Geometry check sheet. Reference: the model listing, model coordinates, mm. Face numbers are marked on the shaded views. Round coordinates to 2 decimals unless told otherwise and drop trailing zeros. Order: outer loops, then holes, each group sorted by start corner. A loop starts at its lowest first (then second) coordinate and runs counter-clockwise, first axis right, second up.
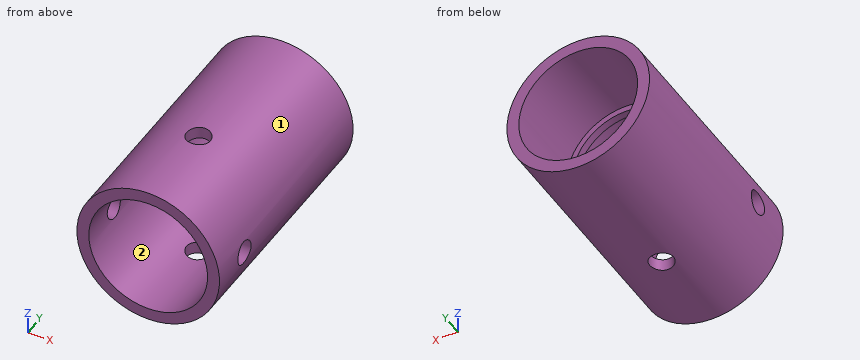
```python
from build123d import *

# Parameters (mm, degrees)
BOSS_EXTRUDE1_DEPTH      = 20
BOSS_EXTRUDE1_DEPTH_BACK = 20
SKETCH1_R                = 9.525
SKETCH1_R_2              = 7.9375
BOSS_EXTRUDE2_DEPTH      = 0.5
BOSS_EXTRUDE2_DEPTH_BACK = 0.5
SKETCH2_R                = 7.9375
SKETCH2_R_2              = 7.178079091
CUT_EXTRUDE1_DEPTH       = 10
CUT_EXTRUDE1_DEPTH_BACK  = 10
SKETCH3_R                = 1.5875
CUT_EXTRUDE2_DEPTH       = 10
CUT_EXTRUDE2_DEPTH_BACK  = 10
SKETCH4_R                = 1.5875
SKETCH5_W                = 27.464518432
SKETCH5_H                = 24.266513238
CUT_EXTRUDE3_DEPTH       = 8


with BuildPart() as part:
    # Sketch1 → Boss-Extrude1 (new, two sides: drawn at the far end of the back side and taken through both)
    with BuildSketch(Plane(origin=(0, 0, 0), x_dir=(1, 0, 0), z_dir=(0, 1, 0)).offset(-BOSS_EXTRUDE1_DEPTH_BACK)):
        with Locations(Location((0, 0, 0), (0, 0, 270))):
            Circle(SKETCH1_R)
        with Locations(Location((0, 0, 0), (0, 0, 270))):
            Circle(SKETCH1_R_2, mode=Mode.SUBTRACT)
    extrude(amount=BOSS_EXTRUDE1_DEPTH + BOSS_EXTRUDE1_DEPTH_BACK)

    # Sketch2 → Boss-Extrude2 (add, two sides: drawn at the far end of the back side and taken through both)
    with BuildSketch(Plane(origin=(0, 0, 0), x_dir=(1, 0, 0), z_dir=(0, 1, 0)).offset(-BOSS_EXTRUDE2_DEPTH_BACK)):
        with Locations(Location((0, 0, 0), (0, 0, 270))):
            Circle(SKETCH2_R)
        with Locations(Location((0, 0, 0), (0, 0, 270))):
            Circle(SKETCH2_R_2, mode=Mode.SUBTRACT)
    extrude(amount=BOSS_EXTRUDE2_DEPTH + BOSS_EXTRUDE2_DEPTH_BACK)

    # Sketch3 → Cut-Extrude1 (cut, two sides: drawn at the far end of the back side and taken through both)
    with BuildSketch(Plane(origin=(0, 0, 0), x_dir=(0, 0, -1), z_dir=(1, 0, 0)).offset(-CUT_EXTRUDE1_DEPTH_BACK)):
        with Locations(Location((0, -14, 0), (0, 0, 180))):
            Circle(SKETCH3_R)
    extrude(amount=CUT_EXTRUDE1_DEPTH + CUT_EXTRUDE1_DEPTH_BACK, mode=Mode.SUBTRACT)

    # Sketch4 → Cut-Extrude2 (cut, two sides: drawn at the far end of the back side and taken through both)
    with BuildSketch(Plane.XY.offset(-CUT_EXTRUDE2_DEPTH_BACK)):
        with Locations(Location((0, -7.965, 0), (0, 0, 180))):
            Circle(SKETCH4_R)
    extrude(amount=CUT_EXTRUDE2_DEPTH + CUT_EXTRUDE2_DEPTH_BACK, mode=Mode.SUBTRACT)

    # Sketch5 → Cut-Extrude3 (cut)
    with BuildSketch(Plane(origin=(0, 20, 0), x_dir=(1, 0, 0), z_dir=(0, 1, 0))):
        Rectangle(SKETCH5_W, SKETCH5_H)
    extrude(amount=-CUT_EXTRUDE3_DEPTH, mode=Mode.SUBTRACT)


solid = part.part
```
(1) Depth check by flat-ended pin: P1, Ø1, axis at y = -4.5, z = -5.5, coming from the +X side; P2, Ø1, axis at y = 1.5, z = 5, coming from the -X side (3 decimals). Enter the tip coordinate at first touch or a pass-through.
Returned:
P1: stops at x = 8.11
P2: stops at x = -8.395
(2) Sectioned sample at B-B, the plane x = 0. Record the cut outline in (y, z) (1 decimal), and give its area (3 significant figures).
Returned:
outline: (-20, -9.5) - (-9.6, -9.5) - (-9.6, -7.9) - (-20, -7.9) - close; (-20, 7.9) - (-9.6, 7.9) - (-9.6, 9.5) - (-20, 9.5) - close; (-6.4, -9.5) - (12, -9.5) - (12, -7.9) - (0.5, -7.9) - (0.5, -7.2) - (-0.5, -7.2) - (-0.5, -7.9) - (-6.4, -7.9) - close; (-6.4, 7.9) - (-0.5, 7.9) - (-0.5, 7.2) - (0.5, 7.2) - (0.5, 7.9) - (12, 7.9) - (12, 9.5) - (-6.4, 9.5) - close
area: 93.0 mm2
(3) Material ranges on line 1 (X direction, y = 7.75, z = 0) (1 decimal); line 2 (X direction, y = -16, z = 5.5); line 3 (Z direction, x = -8.2, y = -14), recorded low to high.
Returned:
line 1: x = -9.5 to -7.9, 7.9 to 9.5
line 2: x = -7.78 to -5.72, 5.72 to 7.78
line 3: z = -4.85 to -1.59, 1.59 to 4.85
(4) Draft check along X on the marked faces 1 and 2. Enter one of: released by +X, released by -X, zero draft, split by the parting line, or undercut.
Returned:
face 1: split by the parting line
face 2: undercut
(5) Sectioned sample at A-A, the plane z = 0. Record the cut outline in (x, y) (1 decimal).
Returned:
outline: (-9.5, -20) - (-7.9, -20) - (-7.9, -15.6) - (-9.5, -15.6) - close; (-9.5, -12.4) - (-7.9, -12.4) - (-7.9, -0.5) - (-7.2, -0.5) - (-7.2, 0.5) - (-7.9, 0.5) - (-7.9, 12) - (-9.5, 12) - close; (7.2, -0.5) - (7.9, -0.5) - (7.9, -12.4) - (9.5, -12.4) - (9.5, 12) - (7.9, 12) - (7.9, 0.5) - (7.2, 0.5) - close; (7.9, -20) - (9.5, -20) - (9.5, -15.6) - (7.9, -15.6) - close
(6) Sectioned sample at D-D, the plane z = -4. Record the cut outline in (x, y), and give its area (3 significant figures).
Returned:
outline: (-8.64, -20) - (-6.86, -20) - (-6.86, -0.5) - (-5.96, -0.5) - (-5.96, 0.5) - (-6.86, 0.5) - (-6.86, 12) - (-8.64, 12) - close; (5.96, -0.5) - (6.86, -0.5) - (6.86, -20) - (8.64, -20) - (8.64, 12) - (6.86, 12) - (6.86, 0.5) - (5.96, 0.5) - close
area: 116 mm2
